Build history of the part. All positions in model axes, mm. A direction names the side the tool comes from. Round coordinates to 2 decimals unless told otherwise and drop trailing zeros. Loops run counter-clockwise (first coordinate to the right, second up) from the corner with the lowest first, then second, coordinate; pieces in that order, holes last. Notation, with made-up numbers: (-6.5, 56) -> (50.5, 56) arc R29 ccw to (50.5, 90) -> close; hole circle Ø8 at (87, 75). An arc over 180 degrees is marked (long way). Put each result on its own line as item: value. Start each with the question number.
Item 1: Tool access for faces 1 (the flat face through (2.4, -0.3, -14.1)), 2 (the flat face through (2.4, 0.3, -14.1)), 3 (the flat face through (-1.4, -2.7, -2.2)), 4 (the flat face through (-3.15, -1, -1)): list every direction of +Z, -Z, +X, -X, +Y, -Y with a clear straight run to the whole face (end or side of a thin tool).
Item 2: Flat gauge pins, fed straight in: pin 1 Ø0.5 at (x, z) = (0, -9) entering from +Y; pin 2 Ø0.5 at (y, z) = (0, -14) entering from +X; pin 3 Ø2 at (y, z) = (-1, -6.5) entering from -X. Where does each tip first touch, or does it go through?
Item 3: Drill centre lines: probe 1 along X at (y, z) = (0.1, -11); probe 2 along Z at (x, y) = (-0.5, 0.7); probe 3 along Y at (x, z) = (-2.25, -2.5). Where is each one in solid material? Low to high. Write a range as [from, to].
Item 4: Cut at D-D, the plane y = -1.25. List the corners of the cut face in (x, z).
Item 5: Cut at C-C, the plane x = -1.25. List the corners of the cut face in (y, z).
Item 6: Cut at A-A, the plane z = -14.75. List the corners of the cut face in (x, y).
Item 7: Cut at B-B, the plane z = 0.5. List the corners of the cut face in (x, y) (3 decimals), plus the area to 3 significant figures.
```python
from build123d import *

# Parameters (mm, degrees)
F1_DEPTH      = 2.7
F1_DEPTH_BACK = 1.4
F0_W          = 0.6
F0_H          = 20
F2_DEPTH      = 0.3


with BuildPart() as f1:
    # F0 (on Front) → F1 (new body, two sides)
    with BuildSketch(Plane.XZ) as f1_sk:
        Polygon((3.15, 2.8), (-3.15, 2.8), (-3.15, -4.2), (-2.2, -4.2), (-1.6, -4.2), (-0.3, -4.2), (0.3, -4.2), (1.6, -4.2), (2.2, -4.2), (3.15, -4.2), align=None)
    extrude(amount=F1_DEPTH)
    extrude(f1_sk.sketch, amount=-F1_DEPTH_BACK)

    # F0 (on Front) → F2 (join, symmetric)
    with BuildSketch(Plane.XZ):
        Polygon((-1.6, -4.2), (-2.2, -4.2), (-2.2, -4.9), (-2.7, -4.9), (-2.7, -24.2), (-2.1, -24.2), (-2.1, -5.6), (-1.6, -5.6), align=None)
        with Locations((0, -14.2)):
            Rectangle(F0_W, F0_H)
        Polygon((2.2, -4.9), (2.2, -4.2), (1.6, -4.2), (1.6, -5.6), (2.1, -5.6), (2.1, -24.2), (2.7, -24.2), (2.7, -4.9), align=None)
    extrude(amount=F2_DEPTH, both=True)

    # F3 (on Top) → F4 (revolve)
    with BuildSketch(Plane.XY):
        with BuildLine():
            ThreePointArc((0, -4.2), (1.3729530218, -3.7918613001), (2.3, -2.7))
            Line((2.3, -2.7), (0, -2.7))
            Line((0, -2.7), (0, -4.2))
        make_face()
    revolve(axis=Axis((0, -4.0003820322, 0), (0, -1, 0)))


solid = f1.part
```
Reply:
1. face 1: -Z, +X, -X, -Y
1. face 2: -Z, +X, -X, +Y
1. face 3: -Y
1. face 4: +Z, -Z, -X, +Y, -Y
2. pin 1: stops at y = 0.3
2. pin 2: stops at x = 2.7
2. pin 3: stops at x = -2.7
3. probe 1: x = [-2.7, -2.1], [-0.3, 0.3], [2.1, 2.7]
3. probe 2: z = [-4.2, 2.8]
3. probe 3: y = [-2.7, 1.4]
4. outline: (-3.15, -4.2) -> (3.15, -4.2) -> (3.15, 2.8) -> (-3.15, 2.8) -> close
5. outline: (-2.7, -4.2) -> (1.4, -4.2) -> (1.4, 2.8) -> (-2.7, 2.8) -> (-2.7, 1.93) arc R2.18 ccw to (-2.7, -1.93) -> close
6. outline: (-2.7, -0.3) -> (-2.1, -0.3) -> (-2.1, 0.3) -> (-2.7, 0.3) -> close; (-0.3, -0.3) -> (0.3, -0.3) -> (0.3, 0.3) -> (-0.3, 0.3) -> close; (2.1, -0.3) -> (2.7, -0.3) -> (2.7, 0.3) -> (2.1, 0.3) -> close
7. outline: (-3.15, -2.7) -> (-2.245, -2.7) arc R2.463 ccw to (2.245, -2.7) -> (3.15, -2.7) -> (3.15, 1.4) -> (-3.15, 1.4) -> close
7. area: 30.5 mm^2
